Verification items for the finished model (mm, model axes). A direction names the side the tool comes from. Round coordinates to 2 decimals unless told otherwise and drop trailing zeros. Order: outer loops, then holes, each group sorted by start corner. A loop starts at its lowest first (then second) coordinate and runs counter-clockwise, first axis right, second up. Notation, with made-up numbers: (37.25, 44) -> (78.25, 44) arc R27 cw to (78.25, 76) -> close; hole circle Ø11 at (7, 21). An arc over 180 degrees is marked (long way). Put each result on its own line as item: value.
Autodesk Inventor part; units mm, degrees
ref_plane "YZ Plane" through (0, 0, 0) normal (1, 0, 0) x (0, 1, 0)
ref_plane "XZ Plane" through (0, 0, 0) normal (0, 1, 0) x (-1, 0, 0)
ref_plane "XY Plane" through (0, 0, 0) normal (0, 0, 1) x (1, 0, 0)
sketch "Sketch1" plane through (0, 0, 0) normal (0, 0, 1) x (1, 0, 0)
  line L0 (10.5, 24.5) -> (-10.5, 24.5)
  line L1 (-10.5, 24.5) -> (-10.5, 35)
  line L2 (10.5, 24.5) -> (10.5, 35)
  line L3 (-10.5, 35) -> (-5, 35)
  line L4 (10.5, 35) -> (5, 35)
  line L5 (2.4732, 27.5) -> (-2.4732, 27.5)
  line L6 (-5, 35) -> (6.4911, 35) construction
  line L7 (5, 35) -> (16.4911, 35) construction
  line L8 (-25.5367, 20) -> (30.733, 20)
  line L9 (-5, 35) -> (-2.4732, 27.5)
  line L10 (2.4732, 27.5) -> (5, 35)
  point P0 (0, 0)
  dimension "d2" = 21
  dimension "d4" = 5.5
  dimension "d5" = 5.5
  dimension "d44" = 9
  dimension "d48" = 15
  dimension "d49" = 30
  dimension "d50" = 30
revolve "Revolution1" add sketch "Sketch1" angle 360 about axis through (-25.5367, 20, 0) along (1, 0, 0)
properties part number "Pulley" material "ABS Plastic"
Item 1: Section check C-C on x = 8.25. Record the boundary of the cut face in (y, z), then the cut area to 3 significant figures.
Check sheet entries:
outline: circle Ø30 at (20, 0); hole circle Ø9 at (20, 0)
area: 643 mm^2
Item 2: Section check D-D on x = 4.25. Record the boundary of the cut face in (y, z).
Check sheet entries:
outline: circle Ø25.55 at (20, 0); hole circle Ø9 at (20, 0)
Item 3: Section check A-A on z = 0. Record the boundary of the cut face in (x, y), then the cut area to 3 significant figures.
Check sheet entries:
outline: (-10.5, 5) -> (-5, 5) -> (-2.47, 12.5) -> (2.47, 12.5) -> (5, 5) -> (10.5, 5) -> (10.5, 15.5) -> (-10.5, 15.5) -> close; (-10.5, 24.5) -> (10.5, 24.5) -> (10.5, 35) -> (5, 35) -> (2.47, 27.5) -> (-2.47, 27.5) -> (-5, 35) -> (-10.5, 35) -> close
area: 329 mm^2
Item 4: Release check for a two-part mould opening along Z. For faces 1 (the flat face through (-10.5, 23, 4)), 2 (the cylindrical face through (-0.147, 15.504, -0.198)), 3 (the cylindrical face through (7.712, 5.015, -0.66)) record: +Z half, -Z half, draft (parallel to the pull), parting line (faces both ways), or undercut.
Check sheet entries:
face 1: draft
face 2: undercut
face 3: parting line
Item 5: Tool access check on faces 4 (the flat face through (10.5, 23, 4)), 5 (the conical face through (-2.63, 27.6, -2.39)). Record the directions out of +Z, -Z, +X, -X, +Y, -Y that give a thin tool (end or side, any length) a straight path to the whole face; none if there is none.
Check sheet entries:
face 4: +Z, -Z, +X, +Y, -Y
face 5: none
Item 6: Material ranges on L1, parallel to Z at x = -6, y = 20; L2, parallel to X at y = 8, z = 6.25; L3, parallel to X at y = 14, z = -8, recorded low to high. Write a range as [from, to].
Check sheet entries:
L1: z = [-15, -4.5], [4.5, 15]
L2: x = [-10.5, -4.5], [4.5, 10.5]
L3: x = [-10.5, -3.32], [3.32, 10.5]
Item 7: Gauge pin test, flat ends, axial feed: pin 1 Ø1 at (y, z) = (16.5, 0.5) entering from +X; pin 2 Ø10 at (x, y) = (5, 28.5) entering from +Z; pin 3 Ø1 at (x, z) = (-7.5, 7.5) entering from +Y; pin 4 Ø6 at (x, z) = (-8, 7.5) entering from +Y. Record the tip position at first contact, or that the pin passes through.
Check sheet entries:
pin 1: passes through
pin 2: stops at z = 14.59
pin 3: stops at y = 33.27
pin 4: stops at y = 34.31
Item 8: Section check B-B on y = 20. Record the boundary of the cut face in (x, z).
Check sheet entries:
outline: (-10.5, -15) -> (-5, -15) -> (-2.47, -7.5) -> (2.47, -7.5) -> (5, -15) -> (10.5, -15) -> (10.5, -4.5) -> (-10.5, -4.5) -> close; (-10.5, 4.5) -> (10.5, 4.5) -> (10.5, 15) -> (5, 15) -> (2.47, 7.5) -> (-2.47, 7.5) -> (-5, 15) -> (-10.5, 15) -> close
